Verification items for the finished model (mm, model axes). A direction names the side the tool comes from. Round coordinates to 2 decimals unless told otherwise and drop trailing zeros. Order: outer loops, then holes, each group sorted by start corner. A loop starts at its lowest first (then second) coordinate and runs counter-clockwise, first axis right, second up. Notation, with made-up numbers: (13, 78.5) -> (30, 78.5) arc R16 ccw to (30, 97.5) -> close; hole circle Ø5 at (50.5, 72). An arc over 180 degrees is marked (long way). Put each result on its own line as item: value.
Autodesk Inventor part; units mm, degrees
ref_plane "YZ Plane" through (0, 0, 0) normal (1, 0, 0) x (0, 1, 0)
ref_plane "XZ Plane" through (0, 0, 0) normal (0, 1, 0) x (-1, 0, 0)
ref_plane "XY Plane" through (0, 0, 0) normal (0, 0, 1) x (1, 0, 0)
sketch "Sketch1" plane through (0, 0, 0) normal (0, 0, 1) x (1, 0, 0)
  line L0 (0, 0) -> (12.7, 0)
  line L1 (0, 0) -> (-12.7, 0)
  circle A0 centre (-12.7, 0) radius 2.3241
  circle A1 centre (12.7, 0) radius 2.3241
  line L2 (-12.7, 0) -> (-6.35, 0)
  circle A2 centre (-12.7, 0) radius 6.35
  circle A3 centre (12.7, 0) radius 6.35
  line L3 (-12.7, -6.35) -> (-10.8231, -6.35)
  line L4 (-10.8231, -6.35) -> (12.7, -6.35)
  line L5 (-19.05, 0) -> (19.05, 0)
  line L6 (19.05, 0) -> (19.05, -50.8)
  line L7 (19.05, -50.8) -> (-19.05, -50.8)
  line L8 (-19.05, -50.8) -> (-19.05, 0)
  line L9 (-6.35, 0) -> (-6.35, -6.35)
  line L10 (6.35, 0) -> (6.35, -6.35)
  dimension "d0" = 12.7
  dimension "d1" = 12.7
  dimension "d2" = 4.6482
  dimension "d3" = 4.6482
  dimension "d5" = 12.7
  dimension "d6" = 50.8
extrude "Extrusion1" add sketch "Sketch1" along normal blind 12.7 contours A3 L5 A1 L0 | L0 A1 L5 A3 | A3 L4 L10 | A2 L5 A0 L1 | L1 A0 L5 A2 | L9 L4 L3 A2 | L6 L7 L8 A2 L3 L4 A3
fillet "Fillet1" radius 3.175 2 edges at (6.35, -6.35, 6.35) (-6.35, -6.35, 6.35)
sketch "Sketch2" plane through (-19.05, -50.8, 0) normal (-1, 0, 0) x (0, 0, 1)
  line L0 (12.7, 50.8) -> (12.7, 0)
  line L1 (0, 0) -> (12.7, 0)
  line L2 (12.7, 0) -> (38.1, 0)
  line L3 (38.1, 0) -> (38.1, 6.35)
  line L4 (38.1, 6.35) -> (12.7, 6.35)
  point P0 (0, 50.8)
  dimension "d10" = 25.4
  dimension "d11" = 6.35
extrude "Extrusion2" add sketch "Sketch2" against normal up to surface (38.1 mm away)
sketch "Sketch3" plane through (-19.05, -44.45, 38.1) normal (0, 1, 0) x (1, 0, 0)
  line L0 (38.1, 0) -> (38.1, 25.4)
  line L1 (0, 25.4) -> (38.1, 25.4)
  line L2 (0, 0) -> (0, 25.4)
  line L3 (0, 0) -> (38.1, 0)
  line L4 (38.1, 0) -> (0, 0)
  line L5 (0, 0) -> (0, 9.525)
  line L6 (0, 9.525) -> (38.1, 9.525)
  line L7 (38.1, 9.525) -> (38.1, 0)
  point P0 (19.05, 38.1)
  dimension "d14" = 9.525
extrude "Extrusion3" add sketch "Sketch3" along normal blind 9.525 contours L3 L2 L6 L0
sketch "Sketch4" plane through (-19.05, -50.8, 0) normal (0, -1, 0) x (1, 0, 0)
  line L0 (0, 0) -> (38.1, 0)
  line L1 (38.1, 0) -> (38.1, 38.1)
  line L2 (0, 38.1) -> (38.1, 38.1)
  line L3 (0, 0) -> (0, 38.1)
  point P0 (19.05, 0)
extrude "Extrusion4" add sketch "Sketch4" along normal blind 3.175
chamfer "Chamfer1" distance 6.35 angle 45 1 edges at (0, -34.925, 38.1)
sketch "Sketch5" plane through (-19.05, 0, 0) normal (-1, 0, 0) x (0, 0, 1)
  line L0 (38.1, -53.975) -> (0, -53.975)
  line L1 (38.1, -53.975) -> (38.1, -52.3875)
  line L2 (38.1, -53.975) -> (38.1, -41.275)
  line L3 (38.1, -52.3875) -> (38.1, -47.7393)
  circle A0 centre (38.1, -47.7393) radius 4.6482
  point P0 (0, 0)
  point P1 (38.1, -43.0911)
  dimension "d22" = 1.5875
  dimension "d23" = 4.6482
extrude "Extrusion5" cut sketch "Sketch5" against normal through all contours A0 L2 picked at (35.7974, -45.6994)
sketch "Sketch6" plane through (-19.05, 0, 0) normal (-1, 0, 0) x (0, 0, 1)
  arc A0 (38.1, -43.0911) -> (38.1, -52.3875) centre (38.1, -47.7393) ccw
  line L0 (38.1, -43.0911) -> (38.1, -41.275)
  line L1 (31.75, -34.925) -> (38.1, -41.275)
  line L2 (28.575, -34.925) -> (31.75, -34.925)
  line L3 (28.575, -44.45) -> (28.575, -34.925)
  line L4 (28.575, -44.45) -> (12.7, -44.45)
  line L5 (12.7, 0) -> (12.7, -44.45)
  line L6 (0, 0) -> (12.7, 0)
  line L7 (0, 0) -> (0, -53.975)
  line L8 (38.1, -53.975) -> (0, -53.975)
  line L9 (38.1, -53.975) -> (38.1, -52.3875)
  line L10 (12.7, -53.975) -> (0, -38.1)
  line L11 (22.617, -46.0414) -> (9.917, -30.1664)
  point P0 (0, 0)
  point P1 (21.3439, -44.45)
  point P2 (12.7, -33.6451)
  dimension "d26" = 12.7
extrude "Extrusion6" cut sketch "Sketch6" against normal through all contours L8 L7 L10
extrude "Extrusion7" add sketch "Sketch6" against normal up to surface (38.1 mm away) contours L4 L5 L11
fillet "Fillet2" radius 12.7 4 edges at (0, -38.1, 0) (0, -53.975, 12.7) (0, -33.6451, 12.7) (0, -44.45, 21.3439)
sketch "Sketch7" plane through (0, 0, 12.7) normal (0, 0, 1) x (1, 0, 0)
  line L0 (19.05, -29.1902) -> (-19.05, -29.1902)
  line L1 (19.05, -29.1902) -> (19.05, 0)
  arc A0 (19.05, 0) -> (6.35, 0) centre (12.7, 0) ccw
  line L2 (6.35, 0) -> (6.35, -3.175)
  arc A1 (3.175, -6.35) -> (6.35, -3.175) centre (3.175, -3.175) ccw
  line L3 (3.175, -6.35) -> (-3.175, -6.35)
  arc A2 (-6.35, -3.175) -> (-3.175, -6.35) centre (-3.175, -3.175) ccw
  line L4 (-6.35, -3.175) -> (-6.35, 0)
  arc A3 (-6.35, 0) -> (-19.05, 0) centre (-12.7, 0) ccw
  line L5 (-19.05, 0) -> (-19.05, -29.1902)
  circle A4 centre (-12.7, 0) radius 2.3241
  circle A5 centre (12.7, 0) radius 2.3241
  line L6 (-3.175, -12.7649) -> (3.175, -12.7649)
  arc A6 (3.175, -12.7649) -> (12.6351, -4.7474) centre (3.175, -3.175) ccw
  line L7 (12.6351, -4.7474) -> (12.6351, -22.7753)
  line L8 (12.6351, -22.7753) -> (-12.6351, -22.7753)
  line L9 (-12.6351, -22.7753) -> (-12.6351, -4.7474)
  arc A7 (-12.6351, -4.7474) -> (-3.175, -12.7649) centre (-3.175, -3.175) ccw
  line L10 (-12.6351, -22.7753) -> (-12.6351, -29.1902)
  line L11 (12.6351, -29.1902) -> (12.6351, -22.7753)
  line L12 (12.6351, -29.1902) -> (-12.6351, -29.1902)
  point P0 (0, 0)
extrude "Extrusion8" cut sketch "Sketch7" against normal through all contours L0 L10 L8 L11 | L8 L9 A7 L6 A6 L7
fillet "Fillet3" radius 3.175 2 edges at (-12.6351, -4.7474, 6.35) (12.6351, -4.7474, 6.35)
fillet "Fillet4" radius 3.175 2 edges at (12.6351, -29.1902, 6.35) (-12.6351, -29.1902, 6.35)
sketch "Sketch8" plane through (-19.05, -34.925, 31.75) normal (0, 0.7071, 0.7071) x (1, 0, 0)
  ellipse E0 centre (31.75, 38.1661) end of major axis (29.4259, 38.1661) minor radius 1.6434
  ellipse E1 centre (6.35, 38.1661) end of major axis (4.0259, 38.1661) minor radius 1.6434
  line L0 (6.4149, 19.7706) -> (6.4149, 28.0648)
  ellipse E2 centre (9.5899, 28.0648) end of major axis (6.4149, 28.0648) minor radius 2.2451 (11.1532, 30.0189) -> (6.4149, 28.0648) ccw
  ellipse E3 centre (15.875, 35.921) end of major axis (25.4649, 35.921) minor radius 6.7811 (11.1532, 30.0189) -> (15.875, 29.1399) ccw
  line L1 (15.875, 29.1399) -> (22.225, 29.1399)
  ellipse E4 centre (22.225, 35.921) end of major axis (12.6351, 35.921) minor radius 6.7811 (22.225, 29.1399) -> (26.9468, 30.0189) ccw
  ellipse E5 centre (28.5101, 28.0648) end of major axis (25.3351, 28.0648) minor radius 2.2451 (31.6851, 28.0648) -> (26.9468, 30.0189) ccw
  line L2 (31.6851, 28.0648) -> (31.6851, 19.7706)
  ellipse E6 centre (28.5101, 19.7706) end of major axis (31.6851, 19.7706) minor radius 2.2451 (28.5101, 17.5255) -> (31.6851, 19.7706) ccw
  line L3 (38.1, 17.5255) -> (28.5101, 17.5255)
  line L4 (38.1, 17.5255) -> (38.1, 38.1661)
  ellipse E7 centre (31.75, 38.1661) end of major axis (38.1, 38.1661) minor radius 4.4901 (38.1, 38.1661) -> (25.4, 38.1661) ccw
  line L5 (25.4, 38.1661) -> (25.4, 35.921)
  ellipse E8 centre (22.225, 35.921) end of major axis (25.4, 35.921) minor radius 2.2451 (22.225, 33.676) -> (25.4, 35.921) ccw
  line L6 (22.225, 33.676) -> (15.875, 33.676)
  ellipse E9 centre (15.875, 35.921) end of major axis (19.05, 35.921) minor radius 2.2451 (12.7, 35.921) -> (15.875, 33.676) ccw
  line L7 (12.7, 35.921) -> (12.7, 38.1661)
  ellipse E10 centre (6.35, 38.1661) end of major axis (12.7, 38.1661) minor radius 4.4901 (12.7, 38.1661) -> (0, 38.1661) ccw
  line L8 (0, 38.1661) -> (0, 17.5255)
  line L9 (9.5899, 17.5255) -> (0, 17.5255)
  ellipse E11 centre (9.5899, 19.7706) end of major axis (12.7649, 19.7706) minor radius 2.2451 (6.4149, 19.7706) -> (9.5899, 17.5255) ccw
  line L10 (6.4149, 17.5255) -> (6.4149, 3.7029)
  line L11 (6.4149, 3.7029) -> (31.75, 4.1664)
  line L12 (31.75, 4.1664) -> (31.75, 17.5255)
  line L13 (6.4149, 17.5255) -> (31.75, 17.5255)
  line L14 (6.4149, 17.5255) -> (6.4149, 12.4851)
  line L15 (6.4149, 12.4851) -> (31.75, 12.4851)
  point P0 (19.05, 47.1463)
extrude "Extrusion9" cut sketch "Sketch8" against normal through all contours L15 L12 L11 L10
properties part number "Rear Jaw"
Item 1: Gauge pin test, flat ends, axial feed: pin 1 Ø3 at (x, z) = (1.5, 9) entering from +Y; pin 2 Ø8 at (x, z) = (-14.5, 7) entering from -Y; pin 3 Ø10 at (x, y) = (12.5, -13.5) entering from +Z; pin 4 Ø1.5 at (x, y) = (-9, -11.5) entering from -Z. Record the tip position at first contact, or that the pin passes through.
Check sheet entries:
pin 1: stops at y = -6.35
pin 2: stops at y = -51.29
pin 3: stops at z = 12.7
pin 4: stops at z = 0
Item 2: Section check A-A on z = 35. Record the boundary of the cut face in (x, y) (3 decimals).
Check sheet entries:
outline: (-19.05, -53.975) -> (19.05, -53.975) -> (19.05, -51.203) -> (-19.05, -51.203) -> close; (-19.05, -44.276) -> (19.05, -44.276) -> (19.05, -38.175) -> (-19.05, -38.175) -> close
Item 3: Section check B-B on x = -7. State how many separate pieces and enclosed holes the cut face has, then the cut area to 3 significant figures.
Check sheet entries:
separate pieces: 3
enclosed holes: 0
area: 615 mm^2
Item 4: Section check D-D on z = 24. Record the boundary of the cut face in (x, y) (3 decimals).
Check sheet entries:
outline: (-19.05, -53.975) -> (19.05, -53.975) -> (19.05, -43.973) -> (-19.05, -43.973) -> close
Item 5: Material ranges on L1, parallel to X at y = 0, z = 2.5; L2, parallel to Z at x = 4, y = -42 (3 decimals); L3, parallel to X at y = -25, z = 7, recorded low to high. Write a range as [from, to].
Check sheet entries:
L1: x = [-19.05, -15.02], [-10.38, -6.35], [6.35, 10.38], [15.02, 19.05]
L2: z = [3.12, 7.018], [19.008, 19.949], [28.575, 38.1]
L3: x = [-19.05, -12.64], [12.64, 19.05]
Item 6: Tool access check on faces 1 (the cylindrical face through (-5.44, -5.4, 6.44)), 2 (the flat face through (12.7, -43, 12)), 3 (the cylindrical face through (0.27, -32.54, 13.15)), 4 (the cylindrical face through (11.73, -28.235, 6.261)). Record the directions out of +Z, -Z, +X, -X, +Y, -Y that give a thin tool (end or side, any length) a straight path to the whole face; none if there is none.
Check sheet entries:
face 1: +Z, -Z, +Y
face 2: none
face 3: +X, -X, +Y
face 4: +Z, -Z
Item 7: Section check C-C on y = -13.5. Record the boundary of the cut face in (x, z).
Check sheet entries:
outline: (-19.05, 0) -> (-12.54, 0) -> (-12.54, 12.7) -> (-19.05, 12.7) -> close; (12.54, 0) -> (19.05, 0) -> (19.05, 12.7) -> (12.54, 12.7) -> close
Item 8: Release check for a two-part mould opening along X. For faces 5 (the flat face through (0, -42, 38.1)), 6 (the cylindrical face through (-5.65, -12.44, 6.44)), 7 (the flat face through (-19.05, -33, 10)), 8 (the flat face through (0, -29.19, 6)) record: +X half, -X half, draft (parallel to the pull), parting line (faces both ways), or undercut.
Check sheet entries:
face 5: draft
face 6: undercut
face 7: -X half
face 8: undercut
